Part model, mm, in its own coordinate system. Face numbers are marked on the shaded views. A direction names the side the tool comes from. Round coordinates to 2 decimals unless told otherwise and drop trailing zeros. Write each loop counter-clockwise with the first axis right and the second up, starting at its lowest first coordinate (ties: lowest second). Pieces come first, ordered by that corner, then holes. Notation, with made-up numbers: (-39.75, 27) -> (-19.75, 27) arc R20 ccw to (-19.75, 49) -> close; hole circle Ø10 at (75, 89). An arc over 180 degrees is marked (long way). Return JSON: item names as keys, results as strings. Group by question number.
(1) Saw through at D-D (z = -236.75). List the corners of the cut face in (x, y), plus the area to 3 significant figures.
(2) Saw through at B-B (z = -225). List the corners of the cut face in (x, y), plus the area to 3 significant figures.
(3) Tool access for the marked faces 1 and 2: list every direction of +Z, -Z, +X, -X, +Y, -Y with a clear straight run to the whole face (end or side of a thin tool).
(4) Drill centre lines: L1, parallel to X at y = 3.5, z = -225; L2, parallel to Z at x = 3, y = 46.5; L3, parallel to X at y = 10, z = -232. Where is each one in solid material? Low to high. Write a range as from..to.
(5) Drop flat-ended pins along their axis: pin 1 Ø3 at (y, z) = (28, -233.5) entering from +X; pin 2 Ø4 at (x, z) = (10.5, -233) entering from +Y; pin 3 Ø5.5 at (y, z) = (46.5, -225) entering from -X; pin 4 Ø6 at (x, z) = (26.5, -221.5) entering from +Y. Give the stop position or say it passes through.
(6) Saw through at A-A (x = 22.5). List the corners of the cut face in (y, z), plus the area to 3 significant figures.
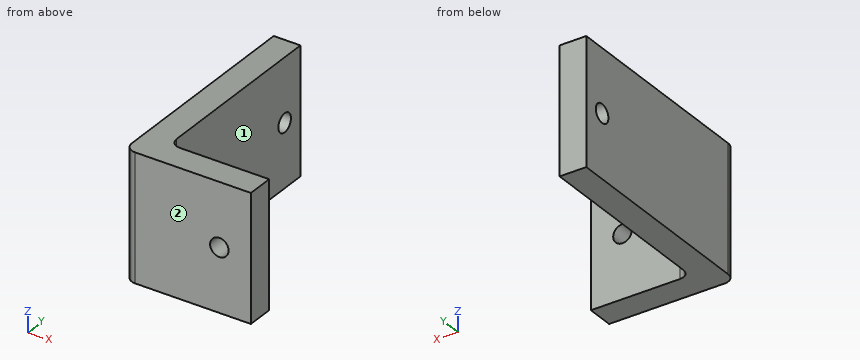
from build123d import *

# Parameters (mm, degrees)
EXTRUDE_THIN1_DEPTH              = 240
SKETCH3_W                        = 35
SKETCH3_H                        = 300
EXTRUDE2_DEPTH                   = 7.35
SKETCH7_W                        = 300
SKETCH7_H                        = 30
EXTRUDE4_DEPTH                   = 7.35
EXTRUDE5_DEPTH                   = 7.35
TAPPED_HOLE_FOR_8_32_HELICOIL1_D = 4.3942
SKETCH26_W                       = 220
SKETCH26_H                       = 70
EXTRUDE18_DEPTH                  = 24.65
EXTRUDE18_DEPTH_BACK             = 7.35
TAPPED_HOLE_FOR_8_32_HELICOIL2_D = 4.3942
FILLET1_R                        = 2.5


with BuildPart() as part:
    # Sketch1 → Extrude-Thin1 (new body)
    with BuildSketch(Plane.XY):
        Polygon((0, 55), (0, 0), (50.8, 0), (50.8, 6.35), (6.35, 6.35), (6.35, 55), align=None)
    extrude(amount=-EXTRUDE_THIN1_DEPTH)

    # Sketch3 → Extrude2 (cut, through all)
    with BuildSketch(Plane(origin=(0, 6.35, 0), x_dir=(1, 0, 0), z_dir=(0, 1, 0))):
        with Locations((47.5, 95)):
            Rectangle(SKETCH3_W, SKETCH3_H)
    extrude(amount=-EXTRUDE2_DEPTH, mode=Mode.SUBTRACT)

    # Sketch7 → Extrude4 (cut, through all)
    with BuildSketch(Plane(origin=(6.35, 0, 0), x_dir=(0, 0, -1), z_dir=(1, 0, 0))):
        with Locations((145, 67)):
            Rectangle(SKETCH7_W, SKETCH7_H)
    extrude(amount=-EXTRUDE4_DEPTH, mode=Mode.SUBTRACT)

    # Sketch10 → Extrude5 (cut, through all)
    with BuildSketch(Plane(origin=(6.35, 0, 0), x_dir=(0, 0, -1), z_dir=(1, 0, 0))):
        with BuildLine():
            Line((30, 67), (210, 67))
            Line((210, 67), (210, 22))
            ThreePointArc((210, 22), (208.535533906, 18.464466094), (205, 17))
            Line((205, 17), (35, 17))
            ThreePointArc((35, 17), (31.464466094, 18.464466094), (30, 22))
            Line((30, 22), (30, 67))
        make_face()
    extrude(amount=-EXTRUDE5_DEPTH, mode=Mode.SUBTRACT)

    # Tapped Hole for #8-32 Helicoil1 (through all)
    with Locations(Plane(origin=(6.35, 46.5, -15), x_dir=(0, 0, 1), z_dir=(1, 0, 0))):
        with Locations((0, 0), (-210, 0)):
            Hole(TAPPED_HOLE_FOR_8_32_HELICOIL1_D / 2)

    # Sketch26 → Extrude18 (cut, two sides)
    with BuildSketch(Plane(origin=(6.35, 0, 0), x_dir=(0, 0, -1), z_dir=(1, 0, 0))) as extrude18_sk:
        with Locations((100, 27)):
            Rectangle(SKETCH26_W, SKETCH26_H)
    extrude(amount=EXTRUDE18_DEPTH, mode=Mode.SUBTRACT)
    extrude(extrude18_sk.sketch, amount=-EXTRUDE18_DEPTH_BACK, mode=Mode.SUBTRACT)

    # Tapped Hole for #8-32 Helicoil2 (through all)
    with Locations(Plane(origin=(22.5, 6.35, -225), x_dir=(0, 0, 1), z_dir=(0, 1, 0))):
        with Locations((0, 0)):
            Hole(TAPPED_HOLE_FOR_8_32_HELICOIL2_D / 2)

    # Fillet1
    fillet1_edges = [part.edges().sort_by_distance(p)[0] for p in [
        (6.35, 6.35, -225),
        (0, 0, -225),
    ]]
    fillet(fillet1_edges, radius=FILLET1_R)


solid = part.part
Computed values:
{
 "1": {"outline": "(0, 2.5) arc R2.5 ccw to (2.5, 0) -> (30, 0) -> (30, 6.35) -> (8.85, 6.35) arc R2.5 cw to (6.35, 8.85) -> (6.35, 52) -> (0, 52) -> close", "area": "480 mm2"},
 "2": {"outline": "(0, 2.5) arc R2.5 ccw to (2.5, 0) -> (20.3, 0) -> (20.3, 6.35) -> (8.85, 6.35) arc R2.5 cw to (6.35, 8.85) -> (6.35, 44.3) -> (0, 44.3) -> close; (0, 48.7) -> (6.35, 48.7) -> (6.35, 52) -> (0, 52) -> close; (24.7, 0) -> (30, 0) -> (30, 6.35) -> (24.7, 6.35) -> close", "area": "425 mm2"},
 "3": {"face 1": "+Z, -Z, +X, +Y", "face 2": "+Z, -Z, +X, -X, -Y"},
 "4": {"L1": "0..20.3, 24.7..30", "L2": "-240..-227.2, -222.8..-210", "L3": "0..6.35"},
 "5": {"pin 1": "x = 6.35", "pin 2": "y = 6.37", "pin 3": "x = 0", "pin 4": "y = 6.35"},
 "6": {"outline": "(0, -240) -> (6.35, -240) -> (6.35, -227.2) -> (0, -227.2) -> close; (0, -222.8) -> (6.35, -222.8) -> (6.35, -210) -> (0, -210) -> close", "area": "163 mm2"}
}
